Study the drawing (mm; zero at the part's minimum x, y, z) and answer. Coordinates: 2 decimals unless noted, no trailing zeros. Order: outer loops, then holes, each group sorted by start corner. A loop starts at its lowest first (then second) coordinate and runs counter-clockwise, first axis right, second up. Notation, with made-up numbers: (18, 34.5) -> (25, 34.5) arc R18 cw to (25, 66.5) -> close; hole circle Ø7 at (-5, 1.5). An arc over 180 degrees is marked (long way). Answer as CSV lines item,"result". Start each with the question number.
Item 1: Section A-A (x = 52.75) is taken. Write down the section's boundary in (y, z).
Item 2: Straight lines are drawn through the part: L1, parallel to X at y = 0.9, z = 15.56; L2, parallel to X at y = 2.45, z = 21.5 (1 decimal); L3, parallel to Z at x = 19.5, y = 2.75 (1 decimal). For each, find the intervals that lie inside material, in ascending order.
Item 3: Section C-C (y = 2.5) is taken. Count the separate pieces of the cut face and the enclosed holes in it, then the cut area to 3 significant figures.
Item 4: Each of these flat-tipped pins is pushed along its axis until it touches: pin 1 Ø1.5 at (y, z) = (1.5, 56) entering from -X; pin 2 Ø1.9 at (x, z) = (52.75, 15.56) entering from -Y; pin 3 Ø1.5 at (y, z) = (2, 52.5) entering from +X. Where does it stop, or does it pass through?
Item 5: Section B-B (z = 55) is taken. Write down the section's boundary in (x, y) (1 decimal).
Item 6: Section D-D (z = 15.56) is taken. Write down the section's boundary in (x, y).
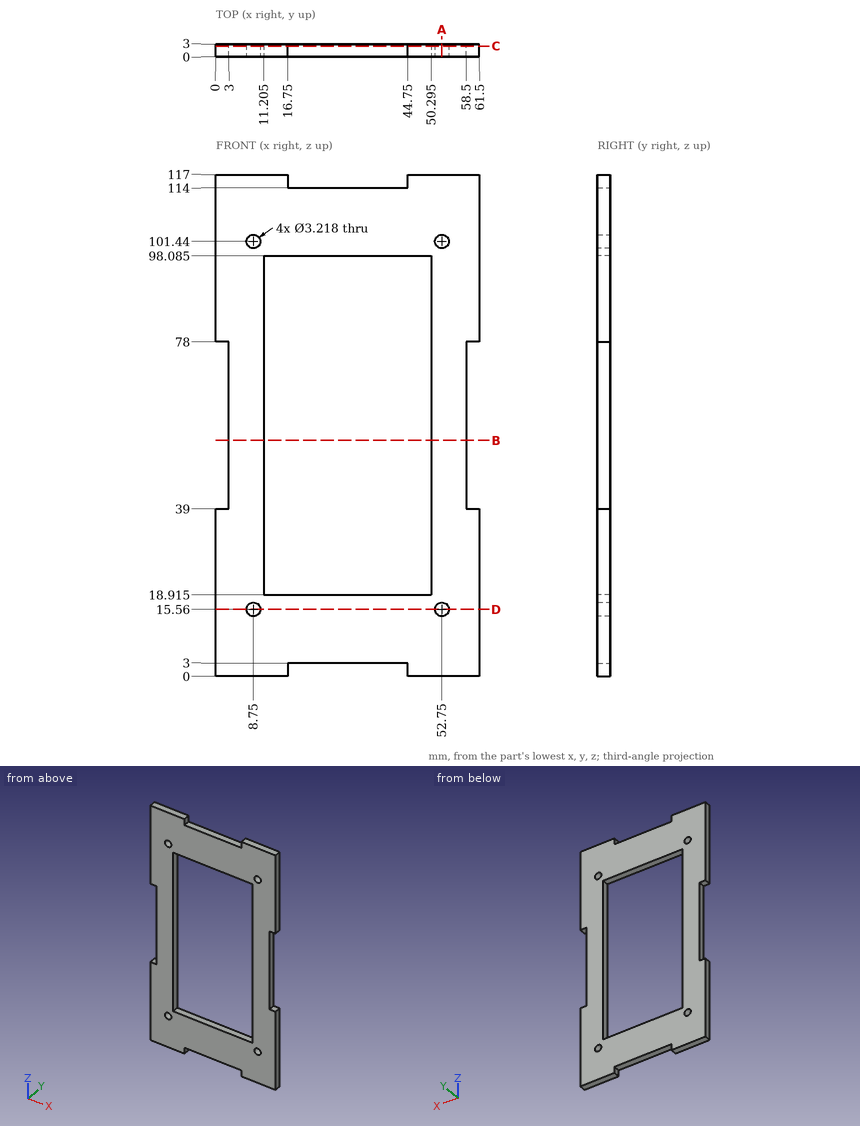
Checked values:
1,outline,"(0, 0) -> (3, 0) -> (3, 13.95) -> (0, 13.95) -> close; (0, 17.17) -> (3, 17.17) -> (3, 99.83) -> (0, 99.83) -> close; (0, 103.05) -> (3, 103.05) -> (3, 117) -> (0, 117) -> close"
2,L1,"x = 0 to 7.14, 10.36 to 51.14, 54.36 to 61.5"
2,L2,"x = 0 to 11.2, 50.3 to 61.5"
2,L3,"z = 3 to 18.9, 98.1 to 114"
3,separate pieces,"1"
3,enclosed holes,"5"
3,area,"3,670 mm^2"
4,pin 1,"stops at x = 3"
4,pin 2,"passes through"
4,pin 3,"stops at x = 58.5"
5,outline,"(3, 0) -> (11.2, 0) -> (11.2, 3) -> (3, 3) -> close; (50.3, 0) -> (58.5, 0) -> (58.5, 3) -> (50.3, 3) -> close"
6,outline,"(0, 0) -> (7.14, 0) -> (7.14, 3) -> (0, 3) -> close; (10.36, 0) -> (51.14, 0) -> (51.14, 3) -> (10.36, 3) -> close; (54.36, 0) -> (61.5, 0) -> (61.5, 3) -> (54.36, 3) -> close"
